Design review of the part built by this model. Coordinates are the model's own, in mm. Coordinates: 2 decimals unless noted, no trailing zeros. Write each loop counter-clockwise with the first axis right and the second up, starting at its lowest first coordinate (ties: lowest second). Pieces come first, ordered by that corner, then holes. Notation, with made-up numbers: (51.25, 7) - (90.25, 7) arc R30 ccw to (90.25, 35) - close; hole circle Ø10 at (33, 41). An arc over 180 degrees is marked (long way). One line per item, written item: value.
from build123d import *

# Parameters (mm, degrees)
SKETCH2_R           = 125
BOSS_EXTRUDE1_DEPTH = 3.18
SKETCH3_R           = 3.5
CUT_EXTRUDE1_DEPTH  = 177.80529517


with BuildPart() as part:
    # Sketch2 → Boss-Extrude1 (new body)
    with BuildSketch(Plane(origin=(0, 0, 0), x_dir=(0, 0, -1), z_dir=(1, 0, 0))):
        with Locations(Location((0, 0, 0), (0, 0, 180))):
            Circle(SKETCH2_R)
    extrude(amount=BOSS_EXTRUDE1_DEPTH)

    # Sketch3 → Cut-Extrude1 (cut, through all)
    with BuildSketch(Plane.ZY):
        with Locations((103.329056078, -15.785012269)):
            Circle(SKETCH3_R)
        with Locations((97.341910159, -39.026227464)):
            Circle(SKETCH3_R)
        with Locations((14.873250681, -103.813680783)):
            Circle(SKETCH3_R)
        with Locations((37.994306415, -97.378093647)):
            Circle(SKETCH3_R)
        with Locations((-65.334749663, -81.593081378)):
            Circle(SKETCH3_R)
        with Locations((-82.468659478, -64.787453318)):
            Circle(SKETCH3_R)
        with Locations((-97.341910159, 39.026227464)):
            Circle(SKETCH3_R)
        with Locations((-103.329056078, 15.785012269)):
            Circle(SKETCH3_R)
        with Locations((-37.994306415, 97.378093647)):
            Circle(SKETCH3_R)
        with Locations((-14.873250681, 103.813680783)):
            Circle(SKETCH3_R)
        with Locations((65.334749663, 81.593081378)):
            Circle(SKETCH3_R)
        with Locations((82.468659478, 64.787453318)):
            Circle(SKETCH3_R)
    extrude(amount=-CUT_EXTRUDE1_DEPTH, mode=Mode.SUBTRACT)


solid = part.part
1. Wall thickness on line 1 along Y through (x, z) = (0.9, 106); line 2 along Z through (x, y) = (1.1, -16); line 3 along Y through (x, z) = (1.45, -3): over which ranges is each line inside the solid? List them lowest first.
Answer block:
line 1: y = -66.25 to -18.05, -13.52 to 66.25
line 2: z = -123.97 to 99.84, 106.82 to 123.97
line 3: y = -124.96 to 124.96
2. Consider section C-C, the plane y = 29.5. Write out the cut boundary in (x, z), then the cut area to 3 significant figures.
Answer block:
outline: (0, -121.47) - (3.18, -121.47) - (3.18, 121.47) - (0, 121.47) - close
area: 773 mm^2
3. Mouldability with a two-part tool opening along Z and no side actions: class faces 1 (the face through (1.57, -5.5, -124.88)), 2 (the face through (3.18, -2, -2)), 3 (the face through (1.57, -67.89, -80.85)) as released by +Z, released by -Z, zero draft, split by the parting line, or undercut.
Answer block:
face 1: split by the parting line
face 2: zero draft
face 3: undercut
4. Consider section A-A, the plane x = 1.2. Give the number of separate pieces and of enclosed holes in the cut face, then the cut area to 3 significant figures.
Answer block:
separate pieces: 1
enclosed holes: 12
area: 48,600 mm^2
5. Insertion check: pin 1 Ø1.5 at (x, z) = (0.5, -52.5) entering from -Y; pin 2 Ø1.5 at (x, z) = (2, -68) entering from -Y. Each pin has a flat end and moves straight along its axis. Give the tip position at first contact, or say it passes through.
Answer block:
pin 1: stops at y = -113.78
pin 2: stops at y = -105.37
6. Consider section B-B, the plane z = -59. Write out the cut boundary in (x, y).
Answer block:
outline: (0, -110.2) - (3.18, -110.2) - (3.18, 110.2) - (0, 110.2) - close
